Could you check a few things on this model? Use its own coordinates, in mm. A direction names the side the tool comes from. Give positions to 0.01 mm unless a question says otherwise; leave off trailing zeros. Loops run counter-clockwise (first coordinate to the right, second up) from the corner with the lowest first, then second, coordinate; pieces in that order, holes last. Notation, with made-up numbers: M -22.75,55 L -10.75,55 A30 cw -10.75,82 Z; hole C -14,-4.75 d5. An arc over 180 degrees is marked long. Use a Markdown table: item, result. Add a question column.
1) Suppose I cut it at C-C on y = 2.5. List the corners of the cut face in (x, z) for me (3 decimals).
2) We'd pull the mould along X, two halves only. Please class faces 3 (the flat face through (0, -12.7, -2)), 4 (the flat face through (0, 9.525, -8)), 5 (the flat face through (12.7, 0, 8)): +X half, -X half, draft (parallel to the pull), parting line (faces both ways), or undercut.
3) Suppose I cut it at D-D on z = 52. List the corners of the cut face in (x, y) for me (3 decimals), and give its area (3 significant figures).
4) Suppose I cut it at B-B on z = -98.5. List the corners of the cut face in (x, y) for me (3 decimals), and give its area (3 significant figures).
5) Suppose I cut it at A-A on x = -3. List the corners of the cut face in (y, z) for me (3 decimals), and give its area (3 significant figures).
6) Which directions (+Z, -Z, +X, -X, +Y, -Y) give clear straight access to the entire face, cutting with the end or side of a thin tool? Please do faces 1 (the flat face through (-9.525, 0, -3)), 2 (the flat face through (10.328, -0.178, -98.6)).
7) If I drill on line 1 along X through (y, z) = (-9.25, 19.5) (3 decimals); line 2 along Z through (x, y) = (-10, -2.25), over which ranges is the centre line in solid material (lowest first)? Write a range as [from, to].
```python
from build123d import *

# Parameters (mm, degrees)
BOSS_EXTRUDE1_DEPTH      = 114.3
BOSS_EXTRUDE1_DEPTH_BACK = 114.3
SKETCH3_W                = 25.4
SKETCH3_H                = 25.4
SKETCH3_W_2              = 19.05
SKETCH3_H_2              = 19.05


with BuildPart() as part:
    # Sketch3 → Boss-Extrude1 (new, two sides: drawn at the far end of the back side and taken through both)
    with BuildSketch(Plane.XY.offset(-BOSS_EXTRUDE1_DEPTH_BACK)):
        Rectangle(SKETCH3_W, SKETCH3_H)
        Rectangle(SKETCH3_W_2, SKETCH3_H_2, mode=Mode.SUBTRACT)
    extrude(amount=BOSS_EXTRUDE1_DEPTH + BOSS_EXTRUDE1_DEPTH_BACK)

    # SurfaceCut2
    split(bisect_by=Plane(origin=(18.506664542, 42.493539826, 75.67626096), x_dir=(0.9713752475559996, 0, -0.2375502650714591), z_dir=(0.20854523863616634, 0.47884508758591265, 0.8527697611530466)), keep=Keep.BOTTOM)

    # SurfaceCut4
    split(bisect_by=Plane(origin=(32.497052155, 0, -7.947169102), x_dir=(0, 1, 0), z_dir=(0.9713752475559998, 0, -0.23755026507145854)), keep=Keep.BOTTOM)


solid = part.part
```
Answer block:
| question | item | result |
|---|---|---|
| 1 | outline | M -12.7,-114.3 L -9.525,-114.3 L -9.525,104.988 L -12.7,105.765 Z; M 9.525,-101.883 L 12.7,-88.9 L 12.7,99.553 L 9.525,100.33 Z |
| 2 | face 3 | draft |
| 2 | face 4 | undercut |
| 2 | face 5 | +X half |
| 3 | outline | M -12.7,-12.7 L 12.7,-12.7 L 12.7,12.7 L -12.7,12.7 Z; hole M -9.525,-9.525 L 9.525,-9.525 L 9.525,9.525 L -9.525,9.525 Z |
| 3 | area | 282 mm^2 |
| 4 | outline | M -12.7,-12.7 L 10.352,-12.7 L 10.352,12.7 L -12.7,12.7 Z; hole M -9.525,-9.525 L 9.525,-9.525 L 9.525,9.525 L -9.525,9.525 Z |
| 4 | area | 223 mm^2 |
| 5 | outline | M -12.7,-114.3 L -9.525,-114.3 L -9.525,110.145 L -12.7,111.928 Z; M 9.525,-114.3 L 12.7,-114.3 L 12.7,97.665 L 9.525,99.448 Z |
| 5 | area | 1,390 mm^2 |
| 6 | face 1 | +Z, -Z |
| 6 | face 2 | -Z, +X, +Y, -Y |
| 7 | line 1 | x = [-12.7, -9.525], [9.525, 12.7] |
| 7 | line 2 | z = [-114.3, 107.77] |
